Could you check a few things on this model? Use its own coordinates, in mm. A direction names the side the tool comes from. Round coordinates to 2 decimals unless told otherwise and drop trailing zeros. Write each loop counter-clockwise with the first axis right and the second up, starting at its lowest first coordinate (ties: lowest second). Pieces come first, ordered by that corner, then holes. Notation, with made-up numbers: (51.25, 19.5) -> (101.25, 19.5) arc R27 cw to (101.25, 48.5) -> close; hole circle Ø7 at (-38.5, -0.5). An arc over 180 degrees is marked (long way). Return JSON: item names as keys, results as strings.
from build123d import *

# Parameters (mm, degrees)
SKETCH1_R           = 2.5527
BOSS_EXTRUDE1_DEPTH = 3.175
FILLET1_R           = 12.7


with BuildPart() as part:
    # Sketch1 → Boss-Extrude1 (new, symmetric)
    # profile 1 of 4: a face of its own
    with BuildSketch(Plane(origin=(0, 0, 0), x_dir=(1, 0, 0), z_dir=(0, 1, 0))):
        with BuildLine():
            Line((25.4, 12.7), (0, 12.7))
            ThreePointArc((0, 12.7), (-12.7, 0), (0, -12.7))
            Line((0, -12.7), (12.7, -12.7))
            Line((12.7, -12.7), (12.7, -2.5527))
            ThreePointArc((12.7, -2.5527), (10.15053309, 0.128435844), (12.95654635, 2.539775829))
            ThreePointArc((12.95654635, 2.539775829), (17.367726132, 9.837305348), (25.4, 12.7))
        make_face()
        with Locations(Location((0, 0, 0), (0, 0, 270))):
            Circle(SKETCH1_R, mode=Mode.SUBTRACT)
    # profile 2 of 4: a face of its own
    with BuildSketch(Plane(origin=(0, 0, 0), x_dir=(1, 0, 0), z_dir=(0, 1, 0))):
        with BuildLine():
            ThreePointArc((37.84345365, 2.539775829), (33.432273868, 9.837305348), (25.4, 12.7))
            ThreePointArc((25.4, 12.7), (17.367726132, 9.837305348), (12.95654635, 2.539775829))
            ThreePointArc((12.95654635, 2.539775829), (14.593563196, 1.711927484), (15.2527, 0))
            ThreePointArc((15.2527, 0), (14.50503148, -1.80503148), (12.7, -2.5527))
            Line((12.7, -2.5527), (12.7, -12.7))
            Line((12.7, -12.7), (22.8473, -12.7))
            ThreePointArc((22.8473, -12.7), (25.4, -10.1473), (27.9527, -12.7))
            Line((27.9527, -12.7), (38.1, -12.7))
            Line((38.1, -12.7), (38.1, -2.5527))
            ThreePointArc((38.1, -2.5527), (35.55053309, -0.128435844), (37.84345365, 2.539775829))
        make_face()
        with Locations(Location((25.4, 0, 0), (0, 0, 270))):
            Circle(SKETCH1_R, mode=Mode.SUBTRACT)
    # profile 3 of 4: a face of its own
    with BuildSketch(Plane(origin=(0, 0, 0), x_dir=(1, 0, 0), z_dir=(0, 1, 0))):
        with BuildLine():
            Line((50.8, 12.7), (25.4, 12.7))
            ThreePointArc((25.4, 12.7), (33.432273868, 9.837305348), (37.84345365, 2.539775829))
            ThreePointArc((37.84345365, 2.539775829), (39.811927484, 1.893563196), (40.6527, 0))
            ThreePointArc((40.6527, 0), (39.90503148, -1.80503148), (38.1, -2.5527))
            Line((38.1, -2.5527), (38.1, -12.7))
            Line((38.1, -12.7), (50.8, -12.7))
            ThreePointArc((50.8, -12.7), (63.5, 0), (50.8, 12.7))
        make_face()
        with Locations(Location((50.8, 0, 0), (0, 0, 270))):
            Circle(SKETCH1_R, mode=Mode.SUBTRACT)
    # profile 4 of 4: a face of its own
    with BuildSketch(Plane(origin=(0, 0, 0), x_dir=(1, 0, 0), z_dir=(0, 1, 0))):
        with BuildLine():
            Line((22.8473, -12.7), (12.7, -12.7))
            Line((12.7, -12.7), (12.7, -38.1))
            ThreePointArc((12.7, -38.1), (25.4, -50.8), (38.1, -38.1))
            Line((38.1, -38.1), (38.1, -12.7))
            Line((38.1, -12.7), (27.9527, -12.7))
            ThreePointArc((27.9527, -12.7), (25.4, -15.2527), (22.8473, -12.7))
        make_face()
        with Locations(Location((25.4, -38.1, 0), (0, 0, 270))):
            Circle(SKETCH1_R, mode=Mode.SUBTRACT)
        with Locations(Location((25.4, -25.4, 0), (0, 0, 270))):
            Circle(SKETCH1_R, mode=Mode.SUBTRACT)
    extrude(amount=BOSS_EXTRUDE1_DEPTH, both=True)

    # Fillet1
    fillet1_edges = [part.edges().sort_by_distance(p)[0] for p in [
        (12.7, 0, 12.7),
        (38.1, 0, 12.7),
    ]]
    fillet(fillet1_edges, radius=FILLET1_R - 0.0001)  # a hair under: the kernel refuses the full size


solid = part.part
1) I want a section at C-C, the plane x = 3.5. Please give me the cut outline in (y, z) (3 decimals), and give its area (3 significant figures).
Return value:
{"outline": "(-3.175, -12.7) -> (3.175, -12.7) -> (3.175, 13.192) -> (-3.175, 13.192) -> close", "area": "164 mm²"}
2) For faces 1 (the face through (25, -3.175, 4)), 2 (the face through (38.1, 0, 32)), 3 (the face through (12.7, 0, 32)), which set-ups out of +Z, -Z, +X, -X, +Y, -Y let a thin tool reach every point of the face, with its end or its side?
Return value:
{"face 1": "+Z, -Z, +X, -X, -Y", "face 2": "+Z, +X, +Y, -Y", "face 3": "+Z, -X, +Y, -Y"}
3) Will these pins go through, and if not, where does the flat tip stop? pin 1 Ø3 at (y, z) = (2, 4) entering from +X; pin 2 Ø3 at (y, z) = (-1, 35) entering from +X; pin 3 Ø1 at (y, z) = (1.5, -4) entering from -X.
Return value:
{"pin 1": "x = 63.25", "pin 2": "x = 38.1", "pin 3": "x = -12.21"}
4) If I drill on probe 1 along X at (y, z) = (-0.5, -1.5); probe 2 along X at (y, z) = (-1.15, 25.4); probe 3 along X at (y, z) = (1, 33), over which ranges is the centre line in solid material (lowest first)? Write a range as [from, to].
Return value:
{"probe 1": "[-12.61, -2.07], [2.07, 10.63], [14.77, 23.33], [27.47, 36.03], [40.17, 48.73], [52.87, 63.41]", "probe 2": "[12.7, 22.85], [27.95, 38.1]", "probe 3": "[12.7, 38.1]"}
5) I want a section at B-B, the plane z = -1. Please give me the cut outline in (x, y) (3 decimals), and give its area (3 significant figures).
Return value:
{"outline": "(-12.661, -3.175) -> (-2.349, -3.175) -> (-2.349, 3.175) -> (-12.661, 3.175) -> close; (2.349, -3.175) -> (10.351, -3.175) -> (10.351, 3.175) -> (2.349, 3.175) -> close; (15.049, -3.175) -> (23.051, -3.175) -> (23.051, 3.175) -> (15.049, 3.175) -> close; (27.749, -3.175) -> (35.751, -3.175) -> (35.751, 3.175) -> (27.749, 3.175) -> close; (40.449, -3.175) -> (48.451, -3.175) -> (48.451, 3.175) -> (40.449, 3.175) -> close; (53.149, -3.175) -> (63.461, -3.175) -> (63.461, 3.175) -> (53.149, 3.175) -> close", "area": "334 mm²"}
6) I want a section at D-D, the plane x = 44.5. Please give me the cut outline in (y, z) (3 decimals), and give its area (3 significant figures).
Return value:
{"outline": "(-3.175, -12.7) -> (3.175, -12.7) -> (3.175, 14.373) -> (-3.175, 14.373) -> close", "area": "172 mm²"}
7) I want a section at A-A, the plane y = 1.5. Count the separate pieces of the cut face and the enclosed holes in it, and give its area (3 significant figures).
Return value:
{"separate pieces": "1", "enclosed holes": "8", "area": "2,600 mm²"}
